Part print with two shaded views. Sizes in mm from the minimum x, y, z corner. A direction names the side the tool comes from. Round coordinates to 2 decimals unless told otherwise and drop trailing zeros. Write each loop counter-clockwise with the first axis right and the second up, starting at its lowest first coordinate (ties: lowest second). Pieces come first, ordered by that corner, then holes. Notation, with made-up numbers: M 76.25,-5 L 105.25,-5 A15 cw 105.25,9 Z; hole C 85,26.25 d6. An arc over 180 degrees is marked long. Use one line per item in the form item = value. Start each with the question number.
Item 1: Cut at C-C, the plane z = 88. Give the cut face in (x, y) (1 decimal), then the cut area to 3 significant figures.
Item 2: Which spindle directions (+Z, -Z, +X, -X, +Y, -Y) get a long thin tool onto all of the face, cutting with end or side? Do the marked faces 1, 2 and 3. Say none if no direction does.
Item 3: Cut at D-D, the plane x = 65.5. Give the cut face in (y, z) (1 decimal), then the cut area to 3 significant figures.
Item 4: Cut at B-B, the plane x = 87.5. Give the cut face in (y, z) (1 decimal), then the cut area to 3 significant figures.
Item 5: Probe L1, parallel to Z at x = 74, y = 107; L2, parallel to X at y = 26, z = 97; L3, parallel to Y at x = 64.5, z = 113 (1 decimal). List the from-to ranges inside material, lowest first.
Item 6: Flat gauge pins, fed straight in: pin 1 Ø20.5 at (y, z) = (29.5, 85) entering from -X; pin 2 Ø1.5 at (y, z) = (102.5, 70) entering from -X. Where does each tip first touch, or does it go through?
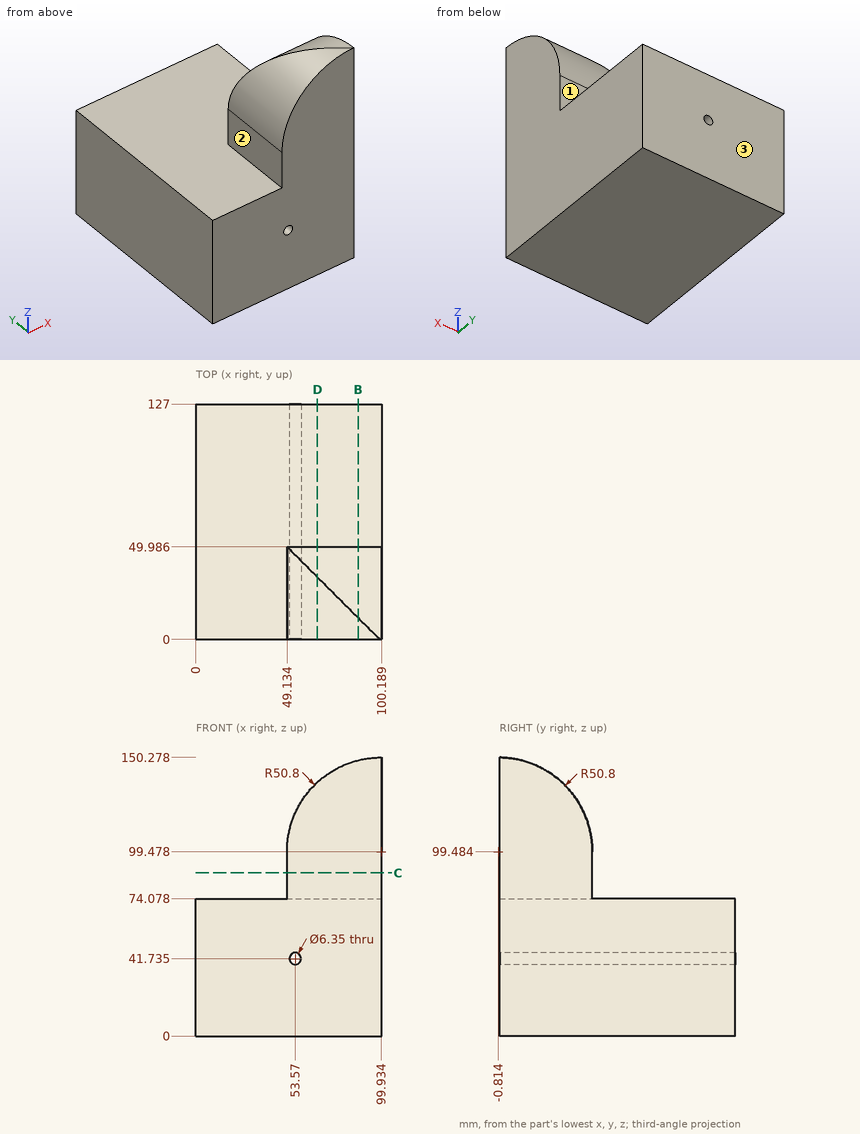
Model answer:
q1.outline = M 49.1,0 L 100.2,0 L 100.2,50 L 49.1,50 Z
q1.area = 2,550 mm²
q2.face_1 = +Z, +X, -X, +Y
q2.face_2 = +Z, -X, +Y, -Y
q2.face_3 = +Z, -Z, +X, -X, +Y
q3.outline = M 0,0 L 127,0 L 127,74.1 L 50,74.1 L 50,99.5 A50.8 ccw 33.6,136.8 L 0,136.8 Z
q3.area = 12,400 mm²
q4.outline = M 0,0 L 127,0 L 127,74.1 L 50,74.1 L 50,99.5 A50.8 ccw 11.6,148.7 L 0,148.7 Z
q4.area = 12,700 mm²
q5.L1 = 0 to 74.08
q5.L2 = 49.13 to 100.19
q5.L3 = 0 to 48.2
q6.pin_1 = 49.13
q6.pin_2 = 0
